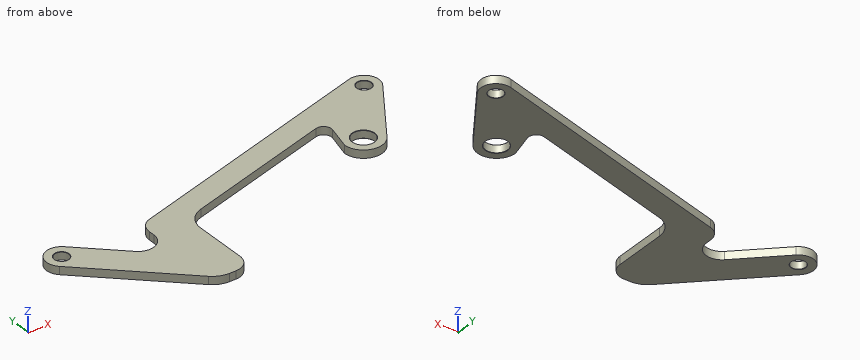
from build123d import *

# Parameters (mm, degrees)
SKETCH1_R           = 6.99
SKETCH1_R_2         = 4.49
BOSS_EXTRUDE1_DEPTH = 5
CHAMFER1_SIZE       = 0.2
CHAMFER2_SIZE       = 0.2
CHAMFER3_SIZE       = 0.2


with BuildPart() as part:
    # Sketch1 → Boss-Extrude1 (new body)
    with BuildSketch(Plane.XY):
        with BuildLine():
            Line((-133.800547442, 2.100285816), (27.342280478, 49.110248457))
            ThreePointArc((27.342280478, 49.110248457), (37.664916823, 45.595457988), (37.867204061, 34.692721954))
            Line((37.867204061, 34.692721954), (9.939702497, -6.705401873))
            ThreePointArc((9.939702497, -6.705401873), (-3.505928341, -11.465974292), (-11.99, 0))
            Line((-11.99, 0), (-8.148421767, 15.289860915))
            ThreePointArc((-8.148421767, 15.289860915), (-9.52943302, 20.109783701), (-14.397978323, 21.308163599))
            Line((-14.397978323, 21.308163599), (-107.124555833, -5.742825892))
            ThreePointArc((-107.124555833, -5.742825892), (-114.923991281, -11.142928518), (-117.92373467, -20.142586361))
            Line((-117.92373467, -20.142586361), (-117.92373467, -53.749229456))
            ThreePointArc((-117.92373467, -53.749229456), (-120.852666858, -60.820297268), (-127.92373467, -63.749229456))
            Line((-127.92373467, -63.749229456), (-131.916457627, -63.749229456))
            ThreePointArc((-131.916457627, -63.749229456), (-137.493140936, -62.674049142), (-142.270365562, -59.602643226))
            Line((-142.270365562, -59.602643226), (-197.550572421, -6.866593112))
            ThreePointArc((-197.550572421, -6.866593112), (-197.866593112, 6.550572421), (-184.449427579, 6.866593112))
            Line((-184.449427579, 6.866593112), (-157.90260529, -18.4584668))
            ThreePointArc((-157.90260529, -18.4584668), (-147.064650772, -20.415954294), (-141, -11.22285762))
            Line((-141, -11.22285762), (-141, -7.499554497))
            ThreePointArc((-141, -7.499554497), (-139.000171074, -1.499782602), (-133.800547442, 2.100285816))
        make_face()
        Circle(SKETCH1_R, mode=Mode.SUBTRACT)
        with Locations((-191, 0)):
            Circle(SKETCH1_R_2, mode=Mode.SUBTRACT)
        with Locations((30, 40)):
            Circle(SKETCH1_R_2, mode=Mode.SUBTRACT)
    extrude(amount=BOSS_EXTRUDE1_DEPTH)

    # Chamfer1
    chamfer1_edges = [part.edges().sort_by_distance(p)[0] for p in [
        (-195.49, 0, 0),
        (-195.49, 0, 5),
    ]]
    chamfer(chamfer1_edges, length=CHAMFER1_SIZE)

    # Chamfer2
    chamfer2_edges = [part.edges().sort_by_distance(p)[0] for p in [
        (-6.99, 0, 0),
        (-6.99, 0, 5),
    ]]
    chamfer(chamfer2_edges, length=CHAMFER2_SIZE)

    # Chamfer3
    chamfer3_edges = [part.edges().sort_by_distance(p)[0] for p in [
        (25.51, 40, 0),
        (25.51, 40, 5),
    ]]
    chamfer(chamfer3_edges, length=CHAMFER3_SIZE)


solid = part.part
For this review, take the finished solid that the model builds, in its own axes (mm). Round coordinates to 2 decimals unless told otherwise and drop trailing zeros. Loops run counter-clockwise (first coordinate to the right, second up) from the corner with the lowest first, then second, coordinate; pieces in that order, holes last. Notation, with made-up numbers: (71.5, -18) - (118.5, -18) arc R16 ccw to (118.5, -5) - close; hole circle Ø11 at (79, -22.5). An arc over 180 degrees is marked (long way). Use one line per item in the form item = value.
Item 1: For line 1 (Y direction, x = 0, z = 3.15); line 2 (Y direction, x = -46.5, z = 3.65); line 3 (X direction, y = -51.5, z = 4.2), list the stretches that pass through material, from the lowest coordinate up.
Answers:
line_1 = -11.99 to -6.99, 6.99 to 41.13
line_2 = 11.94 to 27.57
line_3 = -150.76 to -117.92
Item 2: Consider section C-C on y = 40. Write out the cut boundary in (x, z), then the cut area to 3 significant figures.
Answers:
outline = (-3.89, 0) - (25.31, 0) - (25.51, 0.2) - (25.51, 4.8) - (25.31, 5) - (-3.89, 5) - close; (34.49, 0.2) - (34.69, 0) - (39.49, 0) - (39.49, 5) - (34.69, 5) - (34.49, 4.8) - close
area = 172 mm^2
Item 3: Consider section B-B on x = 0. Write out the cut boundary in (y, z), then the cut area to 3 significant figures.
Answers:
outline = (-11.99, 0) - (-7.19, 0) - (-6.99, 0.2) - (-6.99, 4.8) - (-7.19, 5) - (-11.99, 5) - close; (6.99, 0.2) - (7.19, 0) - (41.13, 0) - (41.13, 5) - (7.19, 5) - (6.99, 4.8) - close
area = 196 mm^2
Item 4: Clearance check with a flat-ended pin moving along its axis: P1, Ø2.5, axis at y = -36.5, z = 2, coming from the +X side. State where the tip first meets the part, or that it passes through.
Answers:
P1 = -117.92
Item 5: Consider section D-D on x = -74. Write out the cut boundary in (y, z).
Answers:
outline = (3.92, 0) - (19.55, 0) - (19.55, 5) - (3.92, 5) - close
Item 6: Consider section A-A on z = 1.55. Write out the cut boundary in (x, y), then the cut area to 3 significant figures.
Answers:
outline = (-197.55, -6.87) - (-142.27, -59.6) arc R15 ccw to (-131.92, -63.75) - (-127.92, -63.75) arc R10 ccw to (-117.92, -53.75) - (-117.92, -20.14) arc R15 cw to (-107.12, -5.74) - (-14.4, 21.31) arc R5 cw to (-8.15, 15.29) - (-11.99, 0) arc R11.99 ccw to (9.94, -6.71) - (37.87, 34.69) arc R9.49 ccw to (27.34, 49.11) - (-133.8, 2.1) arc R10 ccw to (-141, -7.5) - (-141, -11.22) arc R10 cw to (-157.9, -18.46) - (-184.45, 6.87) arc R9.49 ccw to start; hole circle Ø8.98 at (-191, 0); hole circle Ø13.98 at (0, 0); hole circle Ø8.98 at (30, 40)
area = 6,480 mm^2
